```python
from build123d import *

# Parameters (mm, degrees)
F0_R     = 12
F1_DEPTH = 2.75
F2_R     = 4.02
F3_DEPTH = 4
F4_R     = 6.5
F5_DEPTH = 0.5
F6_SIZE  = 0.49999
F7_SIZE  = 1.8
F8_R     = 0.7


# Not quite as in the source:
# - a fillet or chamfer is up to 0.001 mm smaller than in the source, because OpenCascade refuses the exact size


with BuildPart() as f1:
    # F0 (on Top) → F1 (new body)
    with BuildSketch(Plane.XY):
        Circle(F0_R)
    extrude(amount=F1_DEPTH)

    # F2 (on face) → F3 (join)
    with BuildSketch(Plane(origin=(0, 0, 0), x_dir=(1, 0, 0), z_dir=(0, 0, -1))):
        Circle(F2_R)
    extrude(amount=F3_DEPTH)

    # F4 (on face) → F5 (join)
    with BuildSketch(Plane(origin=(0, 0, 0), x_dir=(1, 0, 0), z_dir=(0, 0, -1))):
        Circle(F4_R)
    extrude(amount=F5_DEPTH)

    # F6 (size 0.5 in the source; OpenCascade refuses exactly that, so slightly less here)
    f6_edges = [f1.edges().sort_by_distance(p)[0] for p in [
        (-6.5, 0, -0.5),
        (-4.02, 0, -4),
        (-12, 0, 0),
    ]]
    chamfer(f6_edges, length=F6_SIZE)

    # F7
    f7_edges = [f1.edges().sort_by_distance(p)[0] for p in [
        (-12, 0, 2.75),
    ]]
    chamfer(f7_edges, length=F7_SIZE)

    # F8
    f8_edges = [f1.edges().sort_by_distance(p)[0] for p in [
        (-12, 0, 0.95),
    ]]
    fillet(f8_edges, radius=F8_R)


solid = f1.part
```
The listing builds one solid part. Answer for the finished solid, in the listing's coordinates (mm). A direction names the side the tool comes from. Coordinates: 2 decimals unless noted, no trailing zeros. Write each loop counter-clockwise with the first axis right and the second up, starting at its lowest first coordinate (ties: lowest second). Pieces come first, ordered by that corner, then holes. Notation, with made-up numbers: (39, 88.25) - (78, 88.25) arc R21 cw to (78, 121.25) - close; hole circle Ø10 at (-35.5, -9). An arc over 180 degrees is marked (long way). Return JSON: item names as keys, results as strings. Group by question number.
1. A cutting plane is placed at A-A, the plane z = -2.5. Determine the outline of the cut face in (x, y).
2. Given pin 1 (2 mm diameter, centred on y = 1, z = 2, fed in from -X); pin 2 (4 mm diameter, centred on y = 4.5, z = -0.5, fed in from +X); pin 3 (3 mm diameter, centred on x = -5.5, y = -8, fed in from -Z), each flat-ended and moving along its own axis, determine where each tip first touches the part or whether it passes through.
3. Straight lines are drawn through the part: L1, parallel to Z at x = -6, y = -3; L2, parallel to Z at x = 5, y = 2.5; L3, parallel to Y at x = -6.5, z = 1. For each, find the intervals that lie inside material, in ascending order.
4. Which of the six approach directions +Z, -Z, +X, -X, +Y, -Y give full straight-line access (tool end or side, diameter ignored) to faces 1 (the cylindrical face through (3.834, -1.207, -1.979)), 2 (the flat face through (0, 0, 2.75))?
Ans:
{
 "1": {"outline": "circle Ø8.04 at (0, 0)"},
 "2": {"pin 1": "x = -11.88", "pin 2": "x = 11.68", "pin 3": "z = 0"},
 "3": {"L1": "0 to 2.75", "L2": "-0.5 to 2.75", "L3": "-9.98 to 9.98"},
 "4": {"face 1": "-Z", "face 2": "+Z, +X, -X, +Y, -Y"}
}
